Source: CAD feature listing. Evaluate the final solid. Frame: model axes, mm. Face numbers are marked on the shaded views. A direction names the side the tool comes from. Give positions to 0.01 mm unless a question says otherwise; leave off trailing zeros. Write each loop counter-clockwise with the first axis right and the second up, starting at its lowest first coordinate (ties: lowest second). Pieces come first, ordered by that corner, then holes. Notation, with made-up numbers: (59, -6.5) -> (109, -6.5) arc R18 ccw to (109, 28.5) -> close; hole circle Ø5 at (5, 78.5). An arc over 180 degrees is marked (long way). Write item = value, one per line.
from build123d import *

# Parameters (mm, degrees)
F0_W     = 177.8
F0_H     = 19.05
F2_W     = 20.828
F2_H     = 20.828
F3_DEPTH = 20.828
F6_R     = 9.525
F7_DEPTH = 20.828
F8_SIZE  = 1.524


with BuildPart() as f1:
    # F0 (on Front) → F1 (revolve)
    with BuildSketch(Plane.XZ):
        with Locations((-88.9, 9.525)):
            Rectangle(F0_W, F0_H)
    revolve(axis=Axis((-88.9, 0, 0), (-1, 0, 0)))

    # F2 (on Front) → F3 (cut, symmetric)
    with BuildSketch(Plane.XZ):
        with Locations((-10.414, 10.414)):
            Rectangle(F2_W, F2_H)
    extrude(amount=F3_DEPTH, both=True, mode=Mode.SUBTRACT)

    # F4 (on Front) → F5 (revolve)
    with BuildSketch(Plane.XZ):
        with BuildLine():
            Line((19.05, 0), (0, 0))
            Line((0, 0), (0, -19.05))
            ThreePointArc((0, -19.05), (13.470384, -13.470384), (19.05, 0))
        make_face()
    revolve(axis=Axis((0, 0, -9.525), (0, 0, -1)))

    # F6 (on face) → F7 (join)
    with BuildSketch(Plane.XY):
        Circle(F6_R)
    extrude(amount=F7_DEPTH)

    # F8
    f8_edges = [f1.edges().sort_by_distance(p)[0] for p in [
        (-9.525, 0, 20.828),
    ]]
    chamfer(f8_edges, length=F8_SIZE)


solid = f1.part
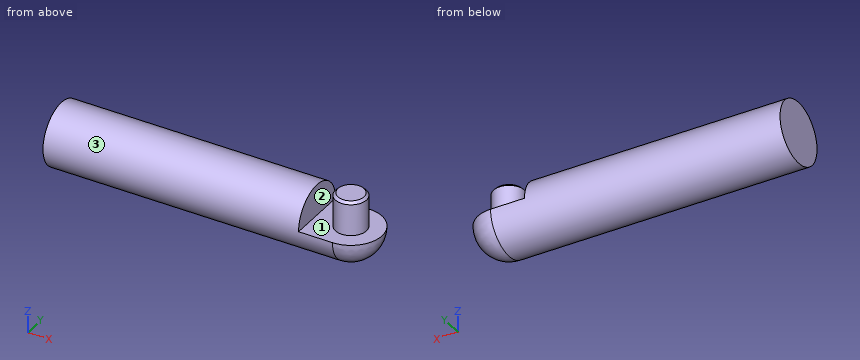
(1) Material intervals for line 1 (X direction, y = 0.5, z = 13.5); line 2 (X direction, y = -15.5, z = 0.5); line 3 (Y direction, x = -21, z = 0.5), sorted ascending.
Values follow:
line_1 = -177.8 to -20.83, -9.51 to 9.51
line_2 = -177.8 to -20.83
line_3 = -19.04 to 19.04
(2) Section query B-B (x = -47). Return loops of the section in (y, z), plus the area to 3 significant figures.
Values follow:
outline = circle Ø38.1 at (0, 0)
area = 1,140 mm2
(3) Access query for the marked faces 1, 2 and 3. Directions: +Z, -Z, +X, -X, +Y, -Y. A direction counts if a zero-diameter tool reaches every point of the face in a straight line with its end or side. Return the directions, or none.
Values follow:
face_1 = +Z
face_2 = +Z, +Y, -Y
face_3 = -X
(4) Section query A-A (z = 12). Return loops of the section in (x, y) (3 decimals), plus the area to 3 significant figures.
Values follow:
outline = (-177.8, -14.795) -> (-20.828, -14.795) -> (-20.828, 14.795) -> (-177.8, 14.795) -> close; circle Ø19.05 at (0, 0)
area = 4,930 mm2
(5) First-contact query: pin 1 (12 mm diameter, centred on y = -9, z = -1.5, fed in from +X); pin 2 (1 mm diameter, centred on x = -55.5, z = 5, fed in from -Y); pin 3 (3 mm diameter, centred on x = -36, z = 9, fed in from +Y). Flat tips, straight axial feed; report the tip coordinate or a pass-through.
Values follow:
pin_1 = 18.79
pin_2 = -18.51
pin_3 = 17.51
